Part print with two shaded views. Sizes in mm from the minimum x, y, z corner. Round coordinates to 2 decimals unless told otherwise and drop trailing zeros. Loops run counter-clockwise (first coordinate to the right, second up) from the corner with the lowest first, then second, coordinate; pieces in that order, holes last.
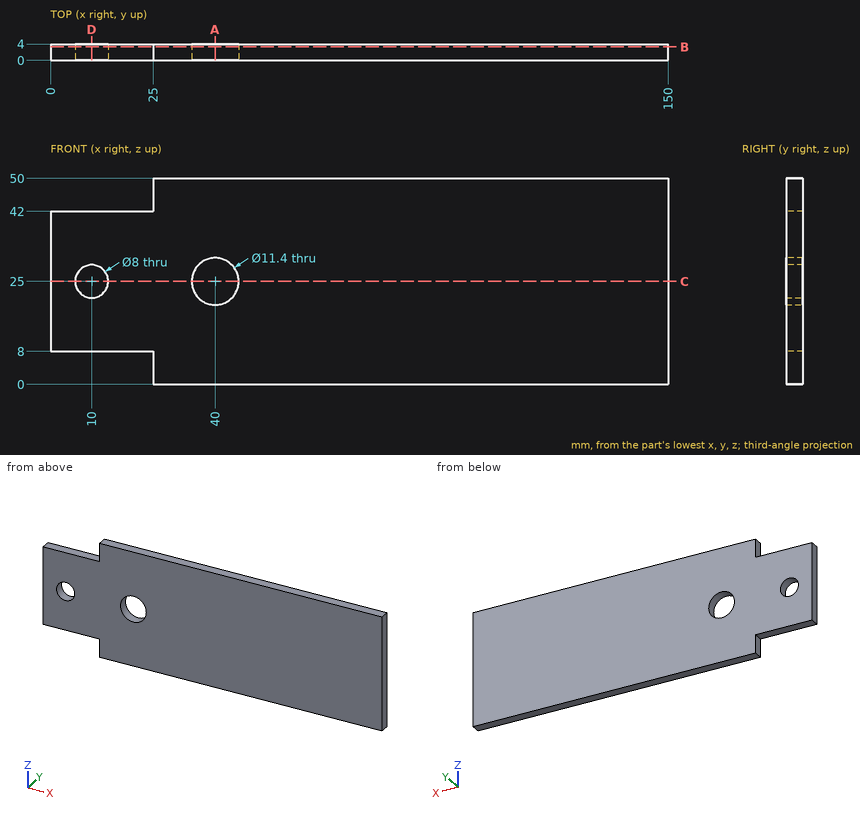
Item 1: Cut at B-B (y = 3.3). List the corners of the cut face in (x, z).
Verdict:
outline: (0, 8) - (25, 8) - (25, 0) - (150, 0) - (150, 50) - (25, 50) - (25, 42) - (0, 42) - close; hole circle Ø8 at (10, 25); hole circle Ø11.4 at (40, 25)
Item 2: Cut at A-A (x = 40). List the corners of the cut face in (y, z), plus the area to 3 significant figures.
Verdict:
outline: (0, 0) - (4, 0) - (4, 19.3) - (0, 19.3) - close; (0, 30.7) - (4, 30.7) - (4, 50) - (0, 50) - close
area: 154 mm2
Item 3: Flat gauge pins, fed straight in: P1, Ø1, axis at x = 117, z = 19.5, coming from the -Y side; P2, Ø2, axis at y = 2, z = 45.5, coming from the -X side; P3, Ø2, axis at x = 14, y = 2.5, coming from the +Z side. Where does each tip first touch, or does it go through?
Verdict:
P1: stops at y = 0
P2: stops at x = 25
P3: stops at z = 42
Item 4: Cut at C-C (z = 25). List the corners of the cut face in (x, y).
Verdict:
outline: (0, 0) - (6, 0) - (6, 4) - (0, 4) - close; (14, 0) - (34.3, 0) - (34.3, 4) - (14, 4) - close; (45.7, 0) - (150, 0) - (150, 4) - (45.7, 4) - close
Item 5: Cut at D-D (x = 10). List the corners of the cut face in (y, z).
Verdict:
outline: (0, 8) - (4, 8) - (4, 21) - (0, 21) - close; (0, 29) - (4, 29) - (4, 42) - (0, 42) - close
Item 6: Wall check: L1, parallel to X at y = 1.65, z = 25; L2, parallel to Z at x = 17, y = 1.6; L3, parallel to X at y = 2.9, z = 46. Give the ranges that are in metal, low to high.
Verdict:
L1: x = 0 to 6, 14 to 34.3, 45.7 to 150
L2: z = 8 to 42
L3: x = 25 to 150
